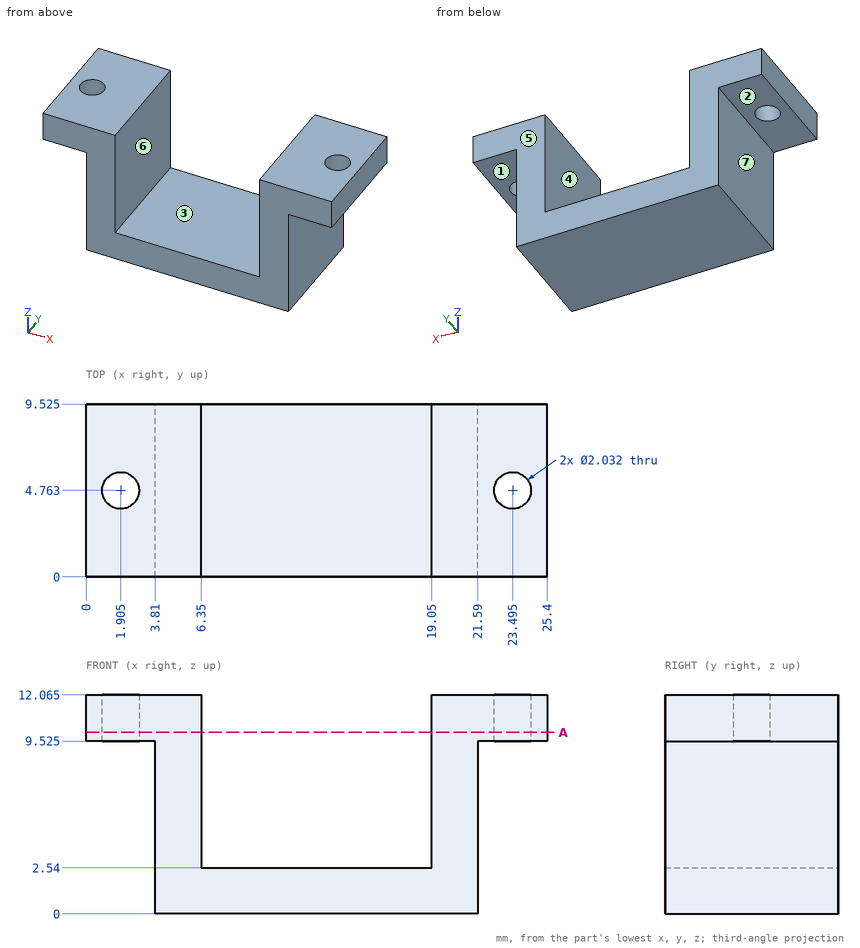
Source: three-view drawing plus pictorial views. Frame: mm from the lowest corner of the part. A direction names the side the tool comes from. Round coordinates to 2 decimals unless told otherwise and drop trailing zeros. Answer as CSV lines item,"result".
Q1. Cut plane A-A (z = 10). Count the separate pieces of the cut face and the enclosed holes in it.
Verdict:
separate pieces,"2"
enclosed holes,"2"
Q2. Pull-direction query (X, two-part tool) for the marked faces 4, 5, 6 and 7; classes: +X half, -X half, draft (parallel to the pull), parting line (faces both ways), or undercut.
Verdict:
face 4,"undercut"
face 5,"draft"
face 6,"undercut"
face 7,"-X half"
Q3. Reachability of the marked faces 1, 2 and 3 from +Z, -Z, +X, -X, +Y, -Y: full face, straight path, thin tool, end or side. Return the list, or none.
Verdict:
face 1,"-Z, +X, +Y, -Y"
face 2,"-Z, -X, +Y, -Y"
face 3,"+Z, +Y, -Y"
Q4. Contact query for flat-ended pins moving along their axis: pin 1 (4 mm diameter, centred on x = 11, y = 7, fed in from +Z); pin 2 (3 mm diameter, centred on y = 4, z = 5.5, fed in from -X); pin 3 (2.5 mm diameter, centred on x = 23.5, y = 4.76, fed in from -Z) (1 decimal). Output: stop coordinate, or through.
Verdict:
pin 1,"stops at z = 2.54"
pin 2,"stops at x = 3.81"
pin 3,"stops at z = 9.5"
Q5. Line query: line 1 along X through (y, z) = (2.5, 8.75); line 2 along X through (y, z) = (1.5, 10); line 3 along Z through (x, y) = (23.5, 8.25) (1 decimal). Output: solid intervals per line, ascending.
Verdict:
line 1,"x = 3.81 to 6.35, 19.05 to 21.59"
line 2,"x = 0 to 6.35, 19.05 to 25.4"
line 3,"z = 9.5 to 12.1"
